from build123d import *

# Parameters (mm, degrees)
BOSS_EXTRUDE1_DEPTH = 34.925


with BuildPart() as part:
    # Sketch1 → Boss-Extrude1 (new body)
    with BuildSketch(Plane(origin=(0, 0, 0), x_dir=(0, 0, -1), z_dir=(1, 0, 0))):
        with BuildLine():
            Line((-4.4069, 8.444220354), (-4.4069, 0))
            Line((-4.4069, 0), (4.4069, 0))
            Line((4.4069, 0), (4.4069, 8.444220354))
            ThreePointArc((4.4069, 8.444220354), (0, 9.525), (-4.4069, 8.444220354))
        make_face()
        with BuildLine():
            Line((4.4069, 0), (-4.4069, 0))
            Line((-4.4069, 0), (-5.2197, 0))
            Line((-5.2197, 0), (-5.2197, 7.967456113))
            ThreePointArc((-5.2197, 7.967456113), (-4.528133307, -8.379834948), (9.525, 0))
            ThreePointArc((9.525, 0), (8.379834948, 4.528133307), (5.2197, 7.967456113))
            Line((5.2197, 7.967456113), (5.2197, 0))
            Line((5.2197, 0), (4.4069, 0))
        make_face()
    extrude(amount=BOSS_EXTRUDE1_DEPTH)


solid = part.part
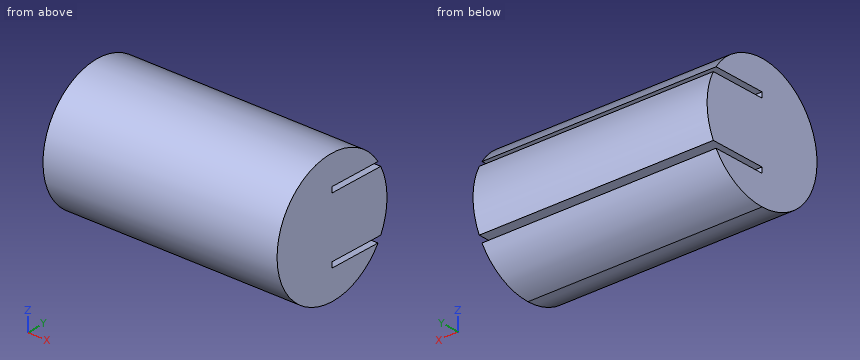
Geometry check sheet. Reference: the model listing, model coordinates, mm. Round coordinates to 2 decimals unless told otherwise and drop trailing zeros. Loops run counter-clockwise (first coordinate to the right, second up) from the corner with the lowest first, then second, coordinate; pieces in that order, holes last. Notation, with made-up numbers: (54, 79.5) - (105, 79.5) arc R27 ccw to (105, 110.5) - close; hole circle Ø5 at (89, 16.25). An arc over 180 degrees is marked (long way). One line per question, with ' | ' between items. Start each with the question number.
1. Cross-section at C-C on z = -7.75. Record the cut outline in (x, y) (3 decimals).
2. Cross-section at D-D on y = -4.75. Record the cut outline in (x, z) (3 decimals), then the cut area to 3 significant figures.
3. Cross-section at A-A on x = 19. Record the cut outline in (y, z) (3 decimals), then the cut area to 3 significant figures.
4. Depth check by flat-ended pin: pin 1 (7 mm diameter, centred on x = 13, y = 6.5, fed in from +Z); pin 2 (6.5 mm diameter, centred on x = 21.5, y = 2.5, fed in from -Z) (3 decimals); pin 3 (4 mm diameter, centred on x = 21.5, z = 3.5, fed in from -Y); pin 4 (3 mm diameter, centred on x = 29.5, z = 3.5, fed in from -Y). Enter the tip coordinate at first touch or a pass-through.
5. Scan lines: line 1 (Z direction, x = 17, y = 2.75); line 2 (Z direction, x = 23.5, y = 5); line 3 (Y direction, x = 15, z = 0) (3 decimals). Record each from-to range of solid material in increasing order. Write a range as [from, to].
6. Cross-section at B-B on y = 6.5. Record the cut outline in (x, z) (3 decimals), then the cut area to 3 significant figures.
Taken from the geometry:
1) outline: (0, -5.537) - (34.925, -5.537) - (34.925, 5.537) - (0, 5.537) - close
2) outline: (0, -8.256) - (34.925, -8.256) - (34.925, 8.256) - (0, 8.256) - close | area: 577 mm²
3) outline: (0, -5.22) - (0, -4.407) - (8.444, -4.407) arc R9.525 ccw to (8.444, 4.407) - (0, 4.407) - (0, 5.22) - (7.967, 5.22) arc R9.525 ccw (long way) to (7.967, -5.22) - close | area: 272 mm²
4) pin 1: z = 9.04 | pin 2: z = -9.525 | pin 3: y = -9.41 | pin 4: y = -9.31
5) line 1: [-9.12, -5.22], [-4.41, 4.41], [5.22, 9.12] | line 2: [-8.11, -5.22], [-4.41, 4.41], [5.22, 8.11] | line 3: [-9.525, 9.525]
6) outline: (0, -6.962) - (34.925, -6.962) - (34.925, -5.22) - (0, -5.22) - close; (0, -4.407) - (34.925, -4.407) - (34.925, 4.407) - (0, 4.407) - close; (0, 5.22) - (34.925, 5.22) - (34.925, 6.962) - (0, 6.962) - close | area: 430 mm²
